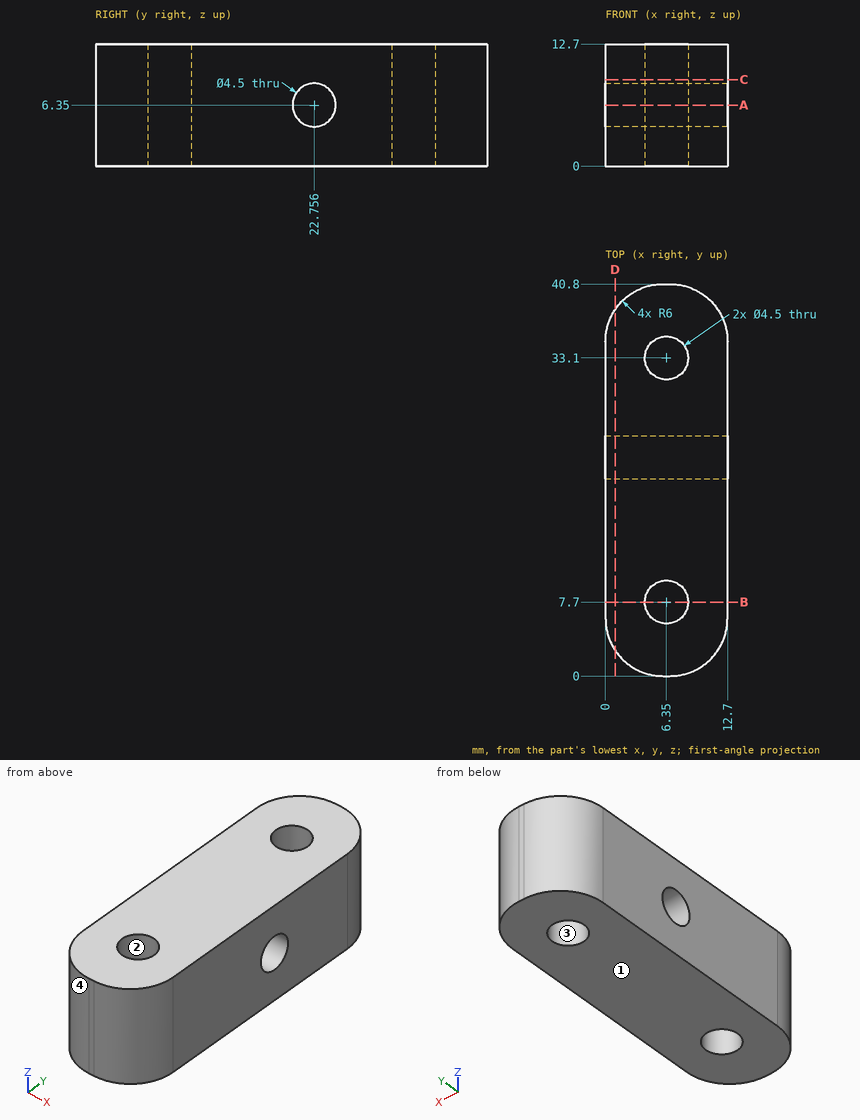
Drawing for the job (mm, zero at the part's lowest x, y, z). Round coordinates to 2 decimals unless told otherwise and drop trailing zeros. Loops run counter-clockwise (first coordinate to the right, second up) from the corner with the lowest first, then second, coordinate; pieces in that order, holes last.
1. Wall check: probe 1 along X at (y, z) = (7.7, 9.5); probe 2 along Y at (x, z) = (6.35, 7); probe 3 along Y at (x, z) = (8, 11.25). Give the ranges that are in metal, low to high.
Check values:
probe 1: x = 0 to 4.1, 8.6 to 12.7
probe 2: y = 0 to 5.45, 9.95 to 20.6, 24.91 to 30.85, 35.35 to 40.8
probe 3: y = 0.14 to 6.17, 9.23 to 31.57, 34.63 to 40.66
2. Band-saw the part on D-D, the plane x = 1. List the corners of the cut face in (y, z).
Check values:
outline: (2.68, 0) - (38.12, 0) - (38.12, 12.7) - (2.68, 12.7) - close; hole circle Ø4.5 at (22.76, 6.35)
3. Mould opens along X. For the marked faces 1, 2, 3 and 4 say: +X half, -X half, draft (parallel to the pull), parting line (faces both ways), or undercut.
Check values:
face 1: draft
face 2: undercut
face 3: undercut
face 4: -X half
4. Band-saw the part on A-A, the plane z = 6.35. List the corners of the cut face in (x, y), and give its area (3 significant figures).
Check values:
outline: (0, 6) arc R6 ccw to (6, 0) - (6.7, 0) arc R6 ccw to (12.7, 6) - (12.7, 20.51) - (0, 20.51) - close; (0, 25.01) - (12.7, 25.01) - (12.7, 34.8) arc R6 ccw to (6.7, 40.8) - (6, 40.8) arc R6 ccw to (0, 34.8) - close; hole circle Ø4.5 at (6.35, 7.7); hole circle Ø4.5 at (6.35, 33.1)
area: 398 mm2
5. Band-saw the part on B-B, the plane y = 7.7. List the corners of the cut face in (x, z), and give its area (3 significant figures).
Check values:
outline: (0, 0) - (4.1, 0) - (4.1, 12.7) - (0, 12.7) - close; (8.6, 0) - (12.7, 0) - (12.7, 12.7) - (8.6, 12.7) - close
area: 104 mm2
6. Band-saw the part on C-C, the plane z = 9. List the corners of the cut face in (x, y).
Check values:
outline: (0, 6) arc R6 ccw to (6, 0) - (6.7, 0) arc R6 ccw to (12.7, 6) - (12.7, 34.8) arc R6 ccw to (6.7, 40.8) - (6, 40.8) arc R6 ccw to (0, 34.8) - close; hole circle Ø4.5 at (6.35, 7.7); hole circle Ø4.5 at (6.35, 33.1)
